Design review of the part built by this model. Coordinates are the model's own, in mm. Round coordinates to 2 decimals unless told otherwise and drop trailing zeros. Loops run counter-clockwise (first coordinate to the right, second up) from the corner with the lowest first, then second, coordinate; pieces in that order, holes last. Notation, with made-up numbers: (-9.75, -12) -> (29.25, -12) arc R29 ccw to (29.25, 20) -> close; hole circle Ø9 at (86, 1.5). An arc over 180 degrees is marked (long way). Answer as CSV lines item,"result". Start each with the question number.
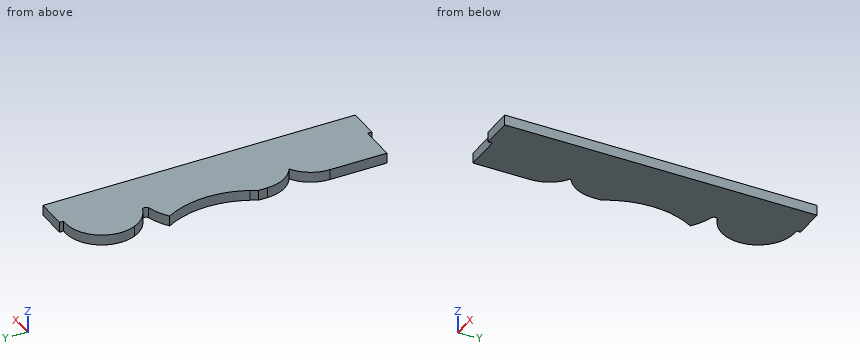
```python
from build123d import *

# Parameters (mm, degrees)
F1_DEPTH = 5


with BuildPart() as f1:
    # F0 (on Top) → F1 (new body)
    with BuildSketch(Plane.XY):
        with BuildLine():
            Line((-17.5, 0), (0, 0))
            Line((0, 0), (0, 128.654855))
            Line((0, 128.654855), (0, 146.075832))
            ThreePointArc((0, 146.075832), (-15.971755, 138.727485), (-17.5, 121.21293))
            ThreePointArc((-17.5, 121.21293), (-13.467707, 115.73757), (-7.652815, 112.212517))
            ThreePointArc((-7.652815, 112.212517), (-6.664225, 110.740832), (-7.762637, 109.349193))
            ThreePointArc((-7.762637, 109.349193), (-12.875909, 107.357911), (-17.5, 104.403503))
            ThreePointArc((-17.5, 104.403503), (-11.796165, 84.899955), (-15.822386, 64.982333))
            ThreePointArc((-15.822386, 64.982333), (-17.075447, 61.336897), (-17.5, 57.505563))
            ThreePointArc((-17.5, 57.505563), (-15.225923, 48.878786), (-8.994711, 42.494061))
            ThreePointArc((-8.994711, 42.494061), (-15.225923, 36.109337), (-17.5, 27.48256))
            Line((-17.5, 27.48256), (-17.5, 0))
        make_face()
        Polygon((0, 128.654855), (0, 0), (0, -2), (15, -2), (15, 148.075832), (0, 148.075832), (0, 146.075832), align=None)
        with BuildLine():
            Line((-17.5, 61.790957), (-17.5, 57.505563))
            ThreePointArc((-17.5, 57.505563), (-17.075447, 61.336897), (-15.822386, 64.982333))
            ThreePointArc((-15.822386, 64.982333), (-16.627255, 63.368805), (-17.5, 61.790957))
        make_face()
    extrude(amount=F1_DEPTH)


solid = f1.part
```
Q1. Add section A-A, the plane x = -13. Give the boundary of the cut face in (y, z), and give its area (3 significant figures).
Q2. Add section B-B, the plane z = 3.7. Give the boundary of the cut face in (x, y), and give its area (3 significant figures).
Q3. To check wall thickness, follow probe 1 along Y at (x, z) = (-10, 4.05); probe 2 along X at (y, z) = (84, 4.2); probe 3 along X at (y, z) = (5.5, 0.75). State the ranges of each line that lie inside material, in increasing order. Write a range as from..to.
Q4. Add section D-D, the plane y = 94. Give the boundary of the cut face in (x, z), and give its area (3 significant figures).
Q5. Add section C-C, the plane y = 59. Give the boundary of the cut face in (x, z), and give its area (4 significant figures).
Q6. For pin 1 Ø1.5 at (y, z) = (44.5, 3) entering from -X; pin 2 Ø1 at (x, z) = (-12.5, 3.5) entering from -Y; pin 3 Ø2.5 at (y, z) = (18, 1.5) entering from -X, all flat-tipped, find the tip position at first contact; note any pin that passes through.
Worked answers:
1,outline,"(0, 0) -> (39.2, 0) -> (39.2, 5) -> (0, 5) -> close; (45.79, 0) -> (72.91, 0) -> (72.91, 5) -> (45.79, 5) -> close; (93.29, 0) -> (107.29, 0) -> (107.29, 5) -> (93.29, 5) -> close; (115.33, 0) -> (141.98, 0) -> (141.98, 5) -> (115.33, 5) -> close"
1,area,"535 mm^2"
2,outline,"(-17.5, 0) -> (0, 0) -> (0, -2) -> (15, -2) -> (15, 148.08) -> (0, 148.08) -> (0, 146.08) arc R17.5 ccw to (-17.5, 121.21) arc R17.5 ccw to (-7.65, 112.21) arc R1.5 cw to (-7.76, 109.35) arc R27.87 ccw to (-17.5, 104.4) arc R42.4 cw to (-15.82, 64.98) arc R42.4 cw to (-17.5, 61.79) -> (-17.5, 57.51) arc R17.5 ccw to (-8.99, 42.49) arc R17.5 ccw to (-17.5, 27.48) -> close"
2,area,"4,460 mm^2"
3,probe 1,"y = 0..41.84, 43.14..108.62, 113.27..144.04"
3,probe 2,"x = -11.77..15"
3,probe 3,"x = -17.5..15"
4,outline,"(-13.18, 0) -> (15, 0) -> (15, 5) -> (-13.18, 5) -> close"
4,area,"141 mm^2"
5,outline,"(-17.5, 0) -> (15, 0) -> (15, 5) -> (-17.5, 5) -> close"
5,area,"162.5 mm^2"
6,pin 1,"stops at x = -12.49"
6,pin 2,"stops at y = 0"
6,pin 3,"stops at x = -17.5"
